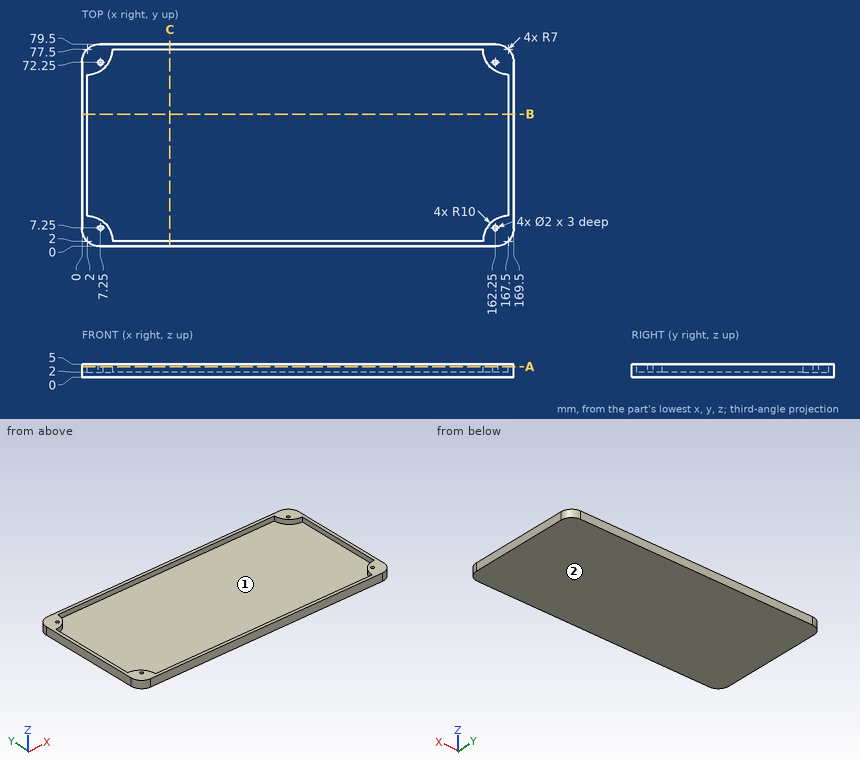
Here's the drawing with two shaded views (mm, measured from the low corner). I have some questions. A direction names the side the tool comes from. Coordinates: 2 decimals unless noted, no trailing zeros. Loops run counter-clockwise (first coordinate to the right, second up) from the corner with the lowest first, then second, coordinate; pieces in that order, holes last. Notation, with made-up numbers: M -25.75,72 L -18.75,72 A18 ccw -18.75,88 Z; hole C 77.5,-29.5 d4. An arc over 180 degrees is marked long. Return JSON: item names as keys, results as strings. Group by question number.
Item 1: Imagine slicing it at A-A (z = 4.1). Please give me the cut outline in (x, y).
Item 2: I'm going to push a flat-ended pin straight in: pin 1 Ø4 at (x, y) = (99, 21) entering from +Z. Where does the tip first touch, or does it pass through?
Item 3: On a 3-axis mill with a long thin cutter (end or side, diameter ignored), from which of +Z, -Z, +X, -X, +Y, -Y can I reach the whole of each face in a straight line? I mean the marked faces 1 and 2. Say none if no direction works.
Item 4: If I drill on L1, parallel to Y at x = 20, z = 4.6; L2, parallel to X at y = 38, z = 2.9; L3, parallel to Y at x = 162.25, z = 3.15, over which ranges is the centre line in solid material (lowest first)? Write a range as from..to.
Item 5: Imagine slicing it at C-C (x = 34.5). Please give me the cut outline in (y, z).
Item 6: Imagine slicing it at B-B (y = 52). Please give me the cut outline in (x, z).
Verdict:
{
 "1": {"outline": "M 0,7 A7 ccw 7,0 L 162.5,0 A7 ccw 169.5,7 L 169.5,72.5 A7 ccw 162.5,79.5 L 7,79.5 A7 ccw 0,72.5 Z; hole M 2,12 A10 cw 12,2 L 157.5,2 A10 cw 167.5,12 L 167.5,67.5 A10 cw 157.5,77.5 L 12,77.5 A10 cw 2,67.5 Z; hole C 7.25,7.25 d2; hole C 7.25,72.25 d2; hole C 162.25,7.25 d2; hole C 162.25,72.25 d2"},
 "2": {"pin 1": "stops at z = 2"},
 "3": {"face 1": "+Z", "face 2": "-Z, +X, -X, +Y, -Y"},
 "4": {"L1": "y = 0..2, 77.5..79.5", "L2": "x = 0..2, 167.5..169.5", "L3": "y = 0..6.25, 8.25..10.51, 68.99..71.25, 73.25..79.5"},
 "5": {"outline": "M 0,0 L 79.5,0 L 79.5,5 L 77.5,5 L 77.5,2 L 2,2 L 2,5 L 0,5 Z"},
 "6": {"outline": "M 0,0 L 169.5,0 L 169.5,5 L 167.5,5 L 167.5,2 L 2,2 L 2,5 L 0,5 Z"}
}
